Could you check a few things on this model? Use its own coordinates, in mm. Face numbers are marked on the shaded views. A direction names the side the tool comes from. Give positions to 0.01 mm unless a question says otherwise; leave off trailing zeros. Write each loop counter-clockwise with the first axis right and the second up, starting at its lowest first coordinate (ties: lowest second). Pieces come first, ordered by that corner, then holes. Notation, with made-up numbers: (-22.75, 72.25) - (23.25, 72.25) arc R19 ccw to (23.25, 103.25) - close; hole circle Ø8 at (44.25, 34.5). An arc over 180 degrees is marked (long way). Write item = value, one per line.
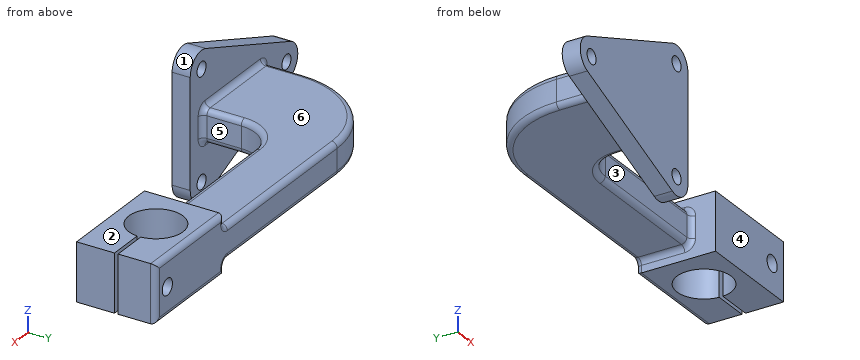
from build123d import *

# Parameters (mm, degrees)
BOSS_EXTRUDE1_DEPTH = 9
SKETCH3_R           = 4
SKETCH3_W           = 55
SKETCH3_H           = 18
BOSS_EXTRUDE2_DEPTH = 10
SKETCH4_W           = 32
SKETCH4_H           = 44
BOSS_EXTRUDE3_DEPTH = 60
SKETCH5_R           = 15
CUT_EXTRUDE1_DEPTH  = 60
SKETCH6_W           = 54.078900839
SKETCH6_H           = 2
CUT_EXTRUDE2_DEPTH  = 60
SKETCH7_R           = 4.5
CUT_EXTRUDE3_DEPTH  = 170.204757616
FILLET1_R           = 3


with BuildPart() as part:
    # Sketch1 → Boss-Extrude1 (new, symmetric)
    with BuildSketch(Plane.XY):
        with BuildLine():
            Line((-112.5, 7.686316473), (-57.5, 7.686316473))
            Line((-57.5, 7.686316473), (-57.5, 29.686316473))
            ThreePointArc((-57.5, 29.686316473), (-51.642135624, 43.828452097), (-37.5, 49.686316473))
            Line((-37.5, 49.686316473), (37.5, 49.686316473))
            Line((37.5, 49.686316473), (37.5, 79.686316473))
            Line((37.5, 79.686316473), (-62.5, 79.686316473))
            ThreePointArc((-62.5, 79.686316473), (-97.855339059, 65.041655533), (-112.5, 29.686316473))
            Line((-112.5, 29.686316473), (-112.5, 7.686316473))
        make_face()
    extrude(amount=BOSS_EXTRUDE1_DEPTH, both=True)

    # Sketch3 → Boss-Extrude2 (add)
    # profile 1 of 2: a face of its own
    with BuildSketch(Plane.XZ.offset(-7.686316473)):
        with BuildLine():
            ThreePointArc((-136.213906764, -9.284766909), (-142.5, 0), (-136.213906764, 9.284766909))
            Line((-136.213906764, 9.284766909), (-61.213906764, 39.284766909))
            ThreePointArc((-61.213906764, 39.284766909), (-51.893711907, 38.280672305), (-47.5, 30))
            Line((-47.5, 30), (-47.5, -30))
            ThreePointArc((-47.5, -30), (-51.893711907, -38.280672305), (-61.213906764, -39.284766909))
            Line((-61.213906764, -39.284766909), (-136.213906764, -9.284766909))
        make_face()
        with Locations(Location((-57.5, 30, 0), (0, 0, 270))):
            Circle(SKETCH3_R, mode=Mode.SUBTRACT)
        with Locations(Location((-57.5, -30, 0), (0, 0, 270))):
            Circle(SKETCH3_R, mode=Mode.SUBTRACT)
        with Locations(Location((-132.5, 0, 0), (0, 0, 270))):
            Circle(SKETCH3_R, mode=Mode.SUBTRACT)
        with Locations((-85, 0)):
            Rectangle(SKETCH3_W, SKETCH3_H, mode=Mode.SUBTRACT)
    # profile 2 of 2: a face of its own
    with BuildSketch(Plane.XZ.offset(-7.686316473)):
        with Locations((-85, 0)):
            Rectangle(SKETCH3_W, SKETCH3_H)
    extrude(amount=BOSS_EXTRUDE2_DEPTH)

    # Sketch4 → Boss-Extrude3 (add)
    with BuildSketch(Plane(origin=(37.5, 0, 0), x_dir=(0, 0, -1), z_dir=(1, 0, 0))):
        with Locations((0, 57.686316473)):
            Rectangle(SKETCH4_W, SKETCH4_H)
    extrude(amount=BOSS_EXTRUDE3_DEPTH)

    # Sketch5 → Cut-Extrude1 (cut)
    with BuildSketch(Plane.XY.offset(16)):
        with Locations((62.5, 57.686316473)):
            Circle(SKETCH5_R)
    extrude(amount=-CUT_EXTRUDE1_DEPTH, mode=Mode.SUBTRACT)

    # Sketch6 → Cut-Extrude2 (cut)
    with BuildSketch(Plane.XY.offset(16)):
        with Locations((94.351130384, 57.686316473)):
            Rectangle(SKETCH6_W, SKETCH6_H)
    extrude(amount=-CUT_EXTRUDE2_DEPTH, mode=Mode.SUBTRACT)

    # Sketch7 → Cut-Extrude3 (cut, through all)
    with BuildSketch(Plane(origin=(0, 79.686316473, 0), x_dir=(1, 0, 0), z_dir=(0, 1, 0))):
        with Locations(Location((87.5, 0, 0), (0, 0, 270))):
            Circle(SKETCH7_R)
    extrude(amount=-CUT_EXTRUDE3_DEPTH, mode=Mode.SUBTRACT)

    # Fillet1
    fillet1_edges = [part.edges().sort_by_distance(p)[0] for p in [
        (-57.5, 18.686316473, 9),
        (-85, 7.686316473, -9),
        (-112.5, 18.686316473, -9),
        (-51.642135624, 43.828452097, 9),
        (37.5, 49.686316473, 0),
        (-57.5, 7.686316473, 0),
        (-112.5, 7.686316473, 0),
        (0, 49.686316473, 9),
        (37.5, 64.686316473, 9),
        (-12.5, 79.686316473, 9),
        (-97.855339059, 65.041655533, 9),
        (-112.5, 18.686316473, 9),
        (97.5, 79.686316473, 0),
        (67.5, 79.686316473, -16),
        (67.5, 79.686316473, 16),
        (37.5, 79.686316473, -12.5),
        (37.5, 79.686316473, 12.5),
        (-85, 7.686316473, 9),
        (-97.855339059, 65.041655533, -9),
        (-12.5, 79.686316473, -9),
        (37.5, 64.686316473, -9),
        (0, 49.686316473, -9),
        (-51.642135624, 43.828452097, -9),
        (-57.5, 18.686316473, -9),
    ]]
    fillet(fillet1_edges, radius=FILLET1_R)


solid = part.part
1. If we section it at B-B, the plane z = 0: Count the separate pieces of the cut face and the enclosed holes in it, and give its area (3 significant figures).
Filled sheet:
separate_pieces = 4
enclosed_holes = 0
area = 8,750 mm2
2. If we section it at C-C, the plane x = 62.5: Please give me the cut outline in (y, z), and give its area (3 significant figures).
Filled sheet:
outline = (35.69, -16) - (42.69, -16) - (42.69, 16) - (35.69, 16) - close; (72.69, -16) - (76.69, -16) arc R3 ccw to (79.69, -13) - (79.69, 13) arc R3 ccw to (76.69, 16) - (72.69, 16) - close
area = 444 mm2
3. If we section it at D-D, the plane y = 24.5: Please give me the cut outline in (x, z), and give its area (3 significant figures).
Filled sheet:
outline = (-112.5, -6) arc R3 ccw to (-109.5, -9) - (-60.5, -9) arc R3 ccw to (-57.5, -6) - (-57.5, 6) arc R3 ccw to (-60.5, 9) - (-109.5, 9) arc R3 ccw to (-112.5, 6) - close
area = 982 mm2
4. For pin 1 (5 mm diameter, centred on x = -41, y = 61, fed in from +Z); pin 2 (9 mm diameter, centred on x = -132.5, z = 0, fed in from +Y); pin 3 (9.5 mm diameter, centred on x = 15.5, z = 2.5, fed in from -Y); pin 4 (13 mm diameter, centred on x = -57.5, z = 30, fed in from -Y), each with a flat end and sliding along its axis, tell me the tip position at first contact or that it passes through.
Filled sheet:
pin_1 = 9
pin_2 = 7.69
pin_3 = 49.69
pin_4 = -2.31
5. Thinking about a two-plate mould opening in X: for the marked faces 1, 2 and 3, which applies, pulls with the +X half, pulls with the -X half, needs draft (parallel to the pull), parting line crosses it, or undercut?
Filled sheet:
face_1 = parting line crosses it
face_2 = needs draft
face_3 = undercut
6. I need wall thicknesses on line 1 (X direction, y = 65, z = 0); line 2 (Y direction, x = 81, z = 9.5); line 3 (X direction, y = 48, z = 0). Which ranges of each line are inside material? Lowest first, please.
Filled sheet:
line_1 = -97.9 to 49.4, 75.6 to 83, 92 to 97.5
line_2 = 35.69 to 56.69, 58.69 to 79.69
line_3 = -109.03 to -45.54, 37.2 to 51.05, 73.95 to 83, 92 to 97.5
7. If we section it at A-A, the plane x = 87.5: Please give me the cut outline in (y, z), and give its area (3 significant figures).
Filled sheet:
outline = (35.69, -16) - (56.69, -16) - (56.69, -4.5) - (35.69, -4.5) - close; (35.69, 4.5) - (56.69, 4.5) - (56.69, 16) - (35.69, 16) - close; (58.69, -16) - (76.69, -16) arc R3 ccw to (79.69, -13) - (79.69, -4.5) - (58.69, -4.5) - close; (58.69, 4.5) - (79.69, 4.5) - (79.69, 13) arc R3 ccw to (76.69, 16) - (58.69, 16) - close
area = 962 mm2
8. Which directions (+Z, -Z, +X, -X, +Y, -Y) give clear straight access to the entire face, cutting with the end or side of a thin tool? Please do the marked faces 4, 5 and 6.
Filled sheet:
face_4 = +Z, -Z, +X, -Y
face_5 = +Z, -Z, +X
face_6 = +Z, -X, +Y
